For this review, use the dimensioned drawing (mm, ordinates from the lowest corner) and the shaded views. A direction names the side the tool comes from. Give positions to 0.01 mm unless a question says otherwise; leave off trailing zeros. Order: outer loops, then holes, each group sorted by start corner. A loop starts at its lowest first (then second) coordinate and runs counter-clockwise, first axis right, second up. Notation, with made-up numbers: (-20, -19) - (-1, -19) arc R27 ccw to (-1, -1) - close; hole circle Ø7 at (69.5, -26). An arc over 180 degrees is marked (long way). Use a Markdown table: item, result. Add a question column.
1) Machinability: for the marked faces 1, 2, 3, 4 and 5, which of the approach directions +Z, -Z, +X, -X, +Y, -Y give a long, thin tool a straight path to every point of the face, cutting with its end or side? Answer none if there is none.
2) We need section C-C on z = 5. Write out the cut boundary in (x, y), then the cut area to 3 significant figures.
3) Wall thickness on L1, parallel to Z at x = 1.25, y = 2.25; L2, parallel to Z at x = 10, y = 3; L3, parallel to X at y = 5, z = 25: over which ranges is each line inside the solid? List them lowest first.
4) We need section B-B on y = 1.75. Write out the cut boundary in (x, z).
5) We need section A-A on x = 4.25. Write out the cut boundary in (y, z).
6) Clearance check with a flat-ended pin moving along its axis: P1, Ø3, axis at y = 3, z = 27.5, coming from the -X side. State where the tip first meets the part, or that it passes through.
7) We need section D-D on x = 6.25. Write out the cut boundary in (y, z).
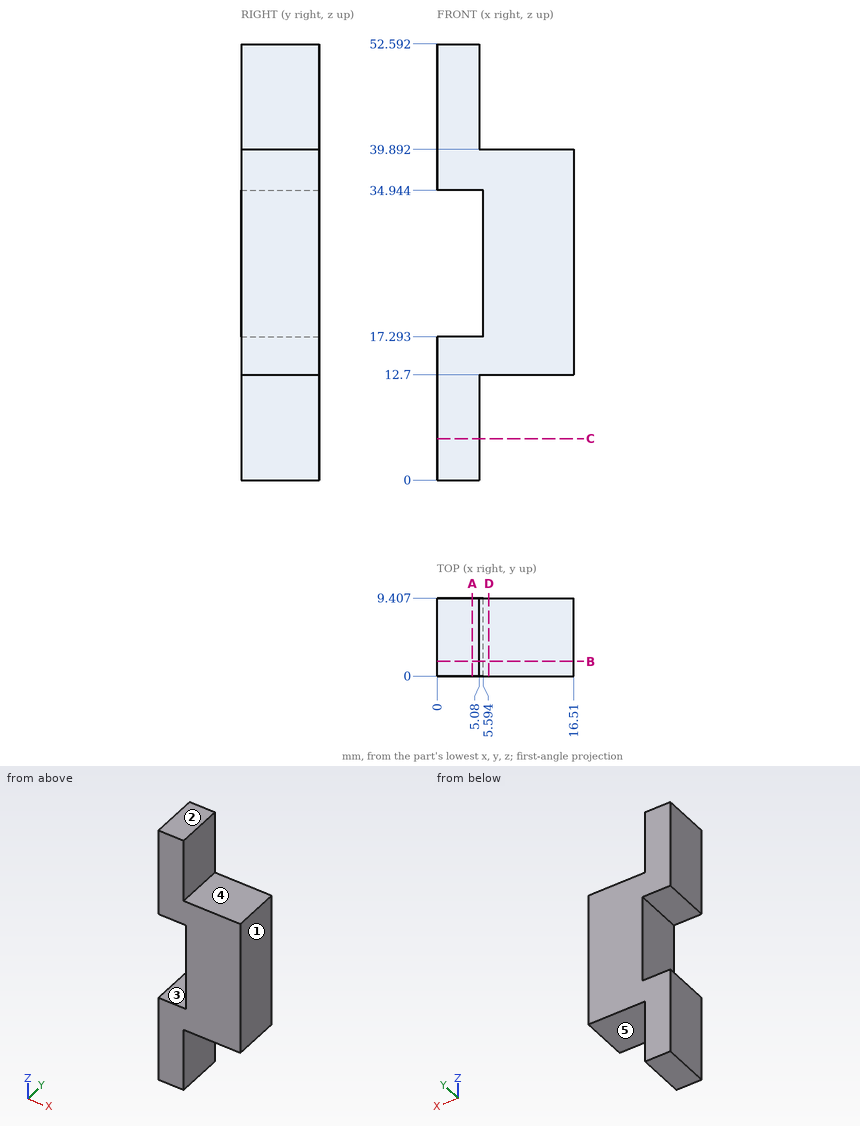
Checked values:
| question | item | result |
|---|---|---|
| 1 | face 1 | +Z, -Z, +X, +Y, -Y |
| 1 | face 2 | +Z, +X, -X, +Y, -Y |
| 1 | face 3 | -X, +Y, -Y |
| 1 | face 4 | +Z, +X, +Y, -Y |
| 1 | face 5 | -Z, +X, +Y, -Y |
| 2 | outline | (0, 0) - (5.08, 0) - (5.08, 9.41) - (0, 9.41) - close |
| 2 | area | 47.8 mm² |
| 3 | L1 | 0 to 17.29, 34.94 to 52.59 |
| 3 | L2 | 12.7 to 39.89 |
| 3 | L3 | 5.59 to 16.51 |
| 4 | outline | (0, 0) - (5.08, 0) - (5.08, 12.7) - (16.51, 12.7) - (16.51, 39.89) - (5.08, 39.89) - (5.08, 52.59) - (0, 52.59) - (0, 34.94) - (5.59, 34.94) - (5.59, 17.29) - (0, 17.29) - close |
| 5 | outline | (0, 0) - (9.41, 0) - (9.41, 17.29) - (0, 17.29) - close; (0, 34.94) - (9.41, 34.94) - (9.41, 52.59) - (0, 52.59) - close |
| 6 | P1 | x = 5.59 |
| 7 | outline | (0, 12.7) - (9.41, 12.7) - (9.41, 39.89) - (0, 39.89) - close |
